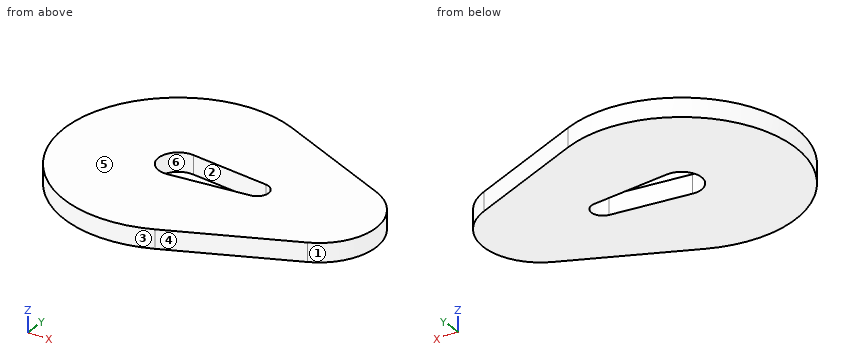
Autodesk Inventor part; units mm, degrees
ref_plane "YZ Plane" through (0, 0, 0) normal (1, 0, 0) x (0, 1, 0)
ref_plane "XZ Plane" through (0, 0, 0) normal (0, 1, 0) x (-1, 0, 0)
ref_plane "XY Plane" through (0, 0, 0) normal (0, 0, 1) x (1, 0, 0)
sketch "Sketch1" plane through (0, 0, 0) normal (0, 0, 1) x (1, 0, 0)
  line L0 (0.3684, -3.4604) -> (14.1917, -1.9888)
  arc A0 (0.3684, 3.4604) -> (0.3684, -3.4604) centre (0, 0) ccw
  line L1 (0.3684, 3.4604) -> (14.1917, 1.9888)
  arc A1 (14.1917, -1.9888) -> (14.1917, 1.9888) centre (13.98, 0) ccw
  line L2 (8, -18.3303) -> (29, -9.1652)
  line L3 (8, 18.3303) -> (29, 9.1652)
  arc A2 (29, -9.1652) -> (29, 9.1652) centre (25, 0) ccw
  arc A3 (8, 18.3303) -> (8, -18.3303) centre (0, 0) ccw
  dimension "d13" = 3.48
  dimension "d14" = 2
  dimension "d15" = 19.46
  dimension "d17" = 20
  dimension "d18" = 10
  dimension "d19" = 25
extrude "Extrusion2" add sketch "Sketch1" along normal blind 3.3
equation "\"d17\" = radio_muslo"
equation "\"d18\" = 0.5 * radio_muslo"
properties part number "Pata - Soporte Antebrazo"
Geometry check sheet. Reference: the model listing, model coordinates, mm. Face numbers are marked on the shaded views. A direction names the side the tool comes from. Round coordinates to 2 decimals unless told otherwise and drop trailing zeros. Loops run counter-clockwise (first coordinate to the right, second up) from the corner with the lowest first, then second, coordinate; pieces in that order, holes last. Notation, with made-up numbers: (81, -6) - (140, -6) arc R19 cw to (140, 10) - close; hole circle Ø5 at (-25, 12). An arc over 180 degrees is marked (long way). Use a Markdown table: item, result.
Q1. Cross-section at C-C on x = 2. Record the cut outline in (y, z).
Solutions:
| item | result |
|---|---|
| outline | (-19.9, 0) - (-3.29, 0) - (-3.29, 3.3) - (-19.9, 3.3) - close; (3.29, 0) - (19.9, 0) - (19.9, 3.3) - (3.29, 3.3) - close |
Q2. Cross-section at D-D on x = -16. Record the cut outline in (y, z).
Solutions:
| item | result |
|---|---|
| outline | (-12, 0) - (12, 0) - (12, 3.3) - (-12, 3.3) - close |
Q3. Go/stop test with flat-tipped pins: P1, Ø1.5, axis at x = 9.5, z = 1.5, coming from the +Y side; P2, Ø1.5, axis at x = -5.5, z = 2, coming from the +Y side. Record where each tip stops, or that it passes through.
Solutions:
| item | result |
|---|---|
| P1 | stops at y = 18 |
| P2 | stops at y = 19.43 |
Q4. Draft check along X on the marked faces 3, 4, 5 and 6. Enter one of: released by +X, released by -X, zero draft, split by the parting line, or undercut.
Solutions:
| item | result |
|---|---|
| face 3 | split by the parting line |
| face 4 | released by +X |
| face 5 | zero draft |
| face 6 | undercut |
Q5. Material ranges on line 1 (Y direction, x = 0, z = 0.7); line 2 (X direction, y = 1.5, z = 2.75); line 3 (Y direction, x = 8, z = 0.75), recorded low to high.
Solutions:
| item | result |
|---|---|
| line 1 | y = -20 to -3.48, 3.48 to 20 |
| line 2 | x = -19.94 to -3.14, 15.3 to 34.89 |
| line 3 | y = -18.33 to -2.65, 2.65 to 18.33 |
Q6. Cross-section at A-A on y = 0. Record the cut outline in (x, z).
Solutions:
| item | result |
|---|---|
| outline | (-20, 0) - (-3.48, 0) - (-3.48, 3.3) - (-20, 3.3) - close; (15.98, 0) - (35, 0) - (35, 3.3) - (15.98, 3.3) - close |
Q7. Access from +Z, -Z, +X, -X, +Y, -Y to the whole of each face (thin tool, end or side, straight path). Record for the marked faces 1 and 2.
Solutions:
| item | result |
|---|---|
| face 1 | +Z, -Z, +X |
| face 2 | +Z, -Z |
Q8. Cross-section at B-B on z = 0.95. Record the cut outline in (x, y).
Solutions:
| item | result |
|---|---|
| outline | (8, -18.33) - (29, -9.17) arc R10 ccw to (29, 9.17) - (8, 18.33) arc R20 ccw (long way) to start; hole (0.37, -3.46) - (14.19, -1.99) arc R2 ccw to (14.19, 1.99) - (0.37, 3.46) arc R3.48 ccw (long way) to start |
